Source: CAD feature listing. Evaluate the final solid. Frame: model axes, mm. A direction names the side the tool comes from. Round coordinates to 2 decimals unless told otherwise and drop trailing zeros. Loops run counter-clockwise (first coordinate to the right, second up) from the corner with the lowest first, then second, coordinate; pieces in that order, holes last. Notation, with made-up numbers: M -37,-16 L -18,-16 A14 cw -18,-12 Z; hole C 77,-39.5 d7. An arc over 180 degrees is marked long. One line per item, written item: value.
from build123d import *

# Parameters (mm, degrees)
SKETCH1_W           = 25
SKETCH1_H           = 25
BOSS_EXTRUDE1_DEPTH = 90
SKETCH2_R           = 4.05
CUT_EXTRUDE1_DEPTH  = 8
SKETCH3_R           = 4.05
CUT_EXTRUDE7_DEPTH  = 8
CHAMFER1_SIZE       = 2
SKETCH5_R           = 1.6
CUT_EXTRUDE8_DEPTH  = 10


with BuildPart() as part:
    # Sketch1 → Boss-Extrude1 (new body)
    with BuildSketch(Plane(origin=(0, 0, 0), x_dir=(1, 0, 0), z_dir=(0, 1, 0))):
        Rectangle(SKETCH1_W, SKETCH1_H)
    extrude(amount=BOSS_EXTRUDE1_DEPTH)

    # Sketch2 → Cut-Extrude1 (cut)
    with BuildSketch(Plane(origin=(12.5, 0, 0), x_dir=(0, 0, -1), z_dir=(1, 0, 0))):
        with Locations((0, 71)):
            Circle(SKETCH2_R)
        with Locations((0, 29)):
            Circle(SKETCH2_R)
    extrude(amount=-CUT_EXTRUDE1_DEPTH, mode=Mode.SUBTRACT)

    # Sketch3 → Cut-Extrude7 (cut)
    with BuildSketch(Plane.XY.offset(12.5)):
        with Locations((0, 29)):
            Circle(SKETCH3_R)
        with Locations((0, 71)):
            Circle(SKETCH3_R)
    extrude(amount=-CUT_EXTRUDE7_DEPTH, mode=Mode.SUBTRACT)

    # Chamfer1
    chamfer1_edges = [part.edges().sort_by_distance(p)[0] for p in [
        (12.5, 45, 12.5),
        (-12.5, 45, 12.5),
        (-12.5, 45, -12.5),
        (12.5, 45, -12.5),
    ]]
    chamfer(chamfer1_edges, length=CHAMFER1_SIZE)

    # Sketch5 → Cut-Extrude8 (cut)
    with BuildSketch(Plane(origin=(0, 90, 0), x_dir=(1, 0, 0), z_dir=(0, 1, 0))):
        Circle(SKETCH5_R)
    extrude(amount=-CUT_EXTRUDE8_DEPTH, mode=Mode.SUBTRACT)


solid = part.part
1. Pin query (flat end, axial travel): pin 1 (4 mm diameter, centred on x = -1, y = 29, fed in from +Z); pin 2 (4 mm diameter, centred on y = 71.5, z = 1.5, fed in from +X); pin 3 (1.9 mm diameter, centred on x = 0, z = 0, fed in from +Y). Return the tip coordinate at first contact, or that it passes through.
Report:
pin 1: stops at z = 4.5
pin 2: stops at x = 4.5
pin 3: stops at y = 80
2. Section query D-D (z = 5.5). Return the cut outline in (x, y), and give its area (3 significant figures).
Report:
outline: M -12.5,0 L 12.5,0 L 12.5,90 L -12.5,90 Z; hole C 0,29 d8.1; hole C 0,71 d8.1
area: 2,150 mm2
3. Section query A-A (x = 7.75). Return the cut outline in (y, z).
Report:
outline: M 0,-12.5 L 90,-12.5 L 90,12.5 L 0,12.5 Z; hole C 29,0 d8.1; hole C 71,0 d8.1
4. Pull-direction query (Y, two-part tool) for faces 4 (the face through (2.2, 74.4, 8.6)), 5 (the face through (0, 80, 0)), 6 (the face through (0, 0, 0)), 7 (the face through (12, 44, 11)); classes: released by +Y, released by -Y, zero draft, split by the parting line, or undercut.
Report:
face 4: undercut
face 5: released by +Y
face 6: released by -Y
face 7: zero draft
5. Ray query, line 1 (Y direction, x = 9.5, z = 0); line 2 (X direction, y = 85.5, z = 0); line 3 (Y direction, x = 10.5, z = -2.75). Return the intervals inside material, ascending. Write a range as [from, to].
Report:
line 1: y = [0, 24.95], [33.05, 66.95], [75.05, 90]
line 2: x = [-12.5, -1.6], [1.6, 12.5]
line 3: y = [0, 26.03], [31.97, 68.03], [73.97, 90]
6. Section query B-B (z = 0). Return the cut outline in (x, y).
Report:
outline: M -12.5,0 L 12.5,0 L 12.5,24.95 L 4.5,24.95 L 4.5,33.05 L 12.5,33.05 L 12.5,66.95 L 4.5,66.95 L 4.5,75.05 L 12.5,75.05 L 12.5,90 L 1.6,90 L 1.6,80 L -1.6,80 L -1.6,90 L -12.5,90 Z
7. Section query C-C (y = 71). Return the cut outline in (x, z), and give its area (3 significant figures).
Report:
outline: M -12.5,-10.5 L -10.5,-12.5 L 10.5,-12.5 L 12.5,-10.5 L 12.5,-4.05 L 4.5,-4.05 L 4.5,4.05 L 12.5,4.05 L 12.5,10.5 L 10.5,12.5 L 4.05,12.5 L 4.05,4.5 L -4.05,4.5 L -4.05,12.5 L -10.5,12.5 L -12.5,10.5 Z
area: 487 mm2
8. Reachability of faces 1 (the face through (8.556, 25.046, 0.878)), 2 (the face through (-1.27, 85.07, 0.97)), 3 (the face through (0, 71, 4.5)) from +Z, -Z, +X, -X, +Y, -Y: full face, straight path, thin tool, end or side. Return the list, or none.
Report:
face 1: +X
face 2: +Y
face 3: +Z
